Work out the finished part from the listing and answer in its coordinate system (mm). Face numbers are marked on the shaded views. A direction names the side the tool comes from. Coordinates: 2 decimals unless noted, no trailing zeros. Order: outer loops, then holes, each group sorted by start corner. A loop starts at its lowest first (then second) coordinate and runs counter-clockwise, first axis right, second up. Notation, with made-up numbers: M -33.75,4 L 7.25,4 A20 cw 7.25,30 Z; hole C -13,0.5 d8. An arc over 180 degrees is marked long. Write item = value, one per line. Start each with the question number.
Q1. Find section B-B on z = -8. Give the vertices of the cut face in (x, y), and give its area (3 significant figures).
Q2. Determine the mould class of the marked faces 1, 2 and 3 for opening direction Z: released by +Z, released by -Z, zero draft, split by the parting line, or undercut.
Q3. Find section C-C on y = 4.5. Give the vertices of the cut face in (x, z).
Q4. Each of these flat-tipped pins is pushed along its axis until it touches: P1, Ø4.5, axis at x = 33, y = 1.5, coming from the -Z side; P2, Ø3, axis at x = 34, y = 2.5, coming from the +Z side; P3, Ø4, axis at y = 6.5, z = -2, coming from the +X side. Where does it stop, or does it pass through?
Q5. Find section A-A on x = 27.8. Give the vertices of the cut face in (y, z).
Q6. Find section D-D on z = -2.8. Give the vertices of the cut face in (x, y), and give its area (3 significant figures).
Q7. Straight lines are drawn through the part: line 1 along X through (y, z) = (1.1, -8); line 2 along X through (y, z) = (3.75, -11); line 3 along X through (y, z) = (5.5, -2.8). For each, find the intervals that lie inside material, in ascending order.
Q8. A tool of negligible diameter and unlimited length cuts with its end or side. For the marked faces 4, 5, 6, 7 and 8, from which of +Z, -Z, +X, -X, +Y, -Y can it reach the whole face along a straight path? Write none if from no direction.
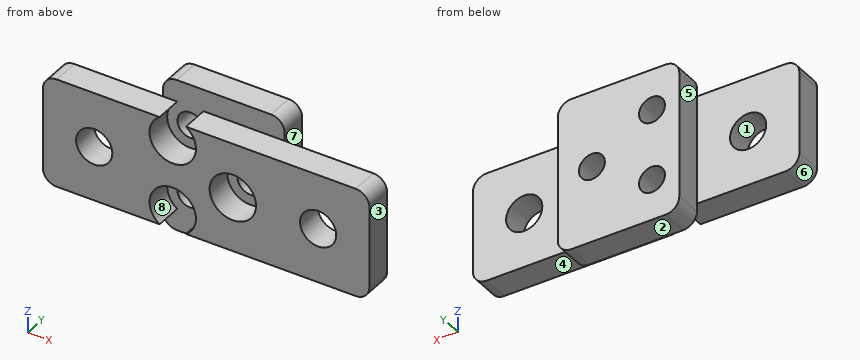
```python
from build123d import *

# Parameters (mm, degrees)
SKETCH1_W           = 47.8
SKETCH1_H           = 16
BOSS_EXTRUDE1_DEPTH = 4
SKETCH2_W           = 17.8
SKETCH2_H           = 22.4
SKETCH2_R           = 1.9
BOSS_EXTRUDE2_DEPTH = 4
SKETCH3_R           = 3.4
CUT_EXTRUDE1_DEPTH  = 4
SKETCH4_R           = 2.65
CUT_EXTRUDE2_DEPTH  = 4
FILLET1_R           = 2


with BuildPart() as part:
    # Sketch1 → Boss-Extrude1 (new body)
    with BuildSketch(Plane(origin=(0, 0, 0), x_dir=(1, 0, 0), z_dir=(0, 1, 0))):
        with Locations((23.9, 8)):
            Rectangle(SKETCH1_W, SKETCH1_H)
    extrude(amount=BOSS_EXTRUDE1_DEPTH)

    # Sketch2 → Boss-Extrude2 (add)
    with BuildSketch(Plane(origin=(0, 4, 0), x_dir=(1, 0, 0), z_dir=(0, 1, 0))):
        with Locations((23.9, 8)):
            Rectangle(SKETCH2_W, SKETCH2_H)
        with Locations(Location((19, 13.2, 0), (0, 0, 270))):
            Circle(SKETCH2_R, mode=Mode.SUBTRACT)
        with Locations(Location((27.8, 8, 0), (0, 0, 270))):
            Circle(SKETCH2_R, mode=Mode.SUBTRACT)
        with Locations(Location((19, 2.8, 0), (0, 0, 270))):
            Circle(SKETCH2_R, mode=Mode.SUBTRACT)
    extrude(amount=BOSS_EXTRUDE2_DEPTH)

    # Sketch3 → Cut-Extrude1 (cut)
    with BuildSketch(Plane.XZ):
        with Locations((19, -2.8)):
            Circle(SKETCH3_R)
        with Locations(Location((27.8, -8, 0), (0, 0, 270))):
            Circle(SKETCH3_R)
        with Locations((19, -13.2)):
            Circle(SKETCH3_R)
    extrude(amount=-CUT_EXTRUDE1_DEPTH, mode=Mode.SUBTRACT)

    # Sketch4 → Cut-Extrude2 (cut)
    with BuildSketch(Plane(origin=(0, 4, 0), x_dir=(1, 0, 0), z_dir=(0, 1, 0))):
        with Locations(Location((7.5, 8, 0), (0, 0, 270))):
            Circle(SKETCH4_R)
        with Locations(Location((40.3, 8, 0), (0, 0, 270))):
            Circle(SKETCH4_R)
    extrude(amount=-CUT_EXTRUDE2_DEPTH, mode=Mode.SUBTRACT)

    # Fillet1
    fillet1_edges = [part.edges().sort_by_distance(p)[0] for p in [
        (15, 6, -19.2),
        (15, 6, 3.2),
        (32.8, 6, 3.2),
        (32.8, 6, -19.2),
        (0, 2, -16),
        (47.8, 2, -16),
        (47.8, 2, 0),
        (0, 2, 0),
    ]]
    fillet(fillet1_edges, radius=FILLET1_R)


solid = part.part
```
Findings below:
q1.outline = M 0,0 L 4.85,0 L 4.85,4 L 0,4 Z; M 10.15,0 L 24.4,0 L 24.4,4 L 25.9,4 L 25.9,8 L 15,8 L 15,4 L 10.15,4 Z; M 29.7,4 L 31.2,4 L 31.2,0 L 37.65,0 L 37.65,4 L 32.8,4 L 32.8,8 L 29.7,8 Z; M 42.95,0 L 47.8,0 L 47.8,4 L 42.95,4 Z
q1.area = 178 mm^2
q2.face_1 = undercut
q2.face_2 = released by -Z
q2.face_3 = zero draft
q3.outline = M 15,-17.2 A2 ccw 17,-19.2 L 30.8,-19.2 A2 ccw 32.8,-17.2 L 32.8,1.2 A2 ccw 30.8,3.2 L 17,3.2 A2 ccw 15,1.2 Z; hole C 19,-13.2 d3.8; hole C 19,-2.8 d3.8; hole C 27.8,-8 d3.8
q4.P1 = -16
q4.P2 = 0
q4.P3 = 32.8
q5.outline = M 0,-16 L 4,-16 L 4,-19.2 L 8,-19.2 L 8,-9.9 L 4,-9.9 L 4,-11.4 L 0,-11.4 Z; M 0,-4.6 L 4,-4.6 L 4,-6.1 L 8,-6.1 L 8,3.2 L 4,3.2 L 4,0 L 0,0 Z
q6.outline = M 0,0 L 15.6,0 L 15.6,4 L 17.1,4 L 17.1,8 L 15,8 L 15,4 L 0,4 Z; M 20.9,4 L 22.4,4 L 22.4,0 L 47.8,0 L 47.8,4 L 32.8,4 L 32.8,8 L 20.9,8 Z
q6.area = 220 mm^2
q7.line_1 = 0 to 4.85, 10.15 to 24.4, 31.2 to 37.65, 42.95 to 47.8
q7.line_2 = 0 to 16.41, 21.59 to 26.2, 29.4 to 47.8
q7.line_3 = 15 to 17.1, 20.9 to 32.8
q8.face_4 = -Z, +X, -X, -Y
q8.face_5 = +Z, -Z, -X, +Y
q8.face_6 = -Z, -X, +Y, -Y
q8.face_7 = +Z, -Z, +X, +Y
q8.face_8 = -Y
